Read the model definition and answer for the solid it produces. Units are mm, in the model's axes. Face numbers are marked on the shaded views. A direction names the side the tool comes from. Coordinates: 2 decimals unless noted, no trailing zeros. Write each loop counter-clockwise with the first axis right and the second up, starting at its lowest first coordinate (ties: lowest second). Pieces come first, ordered by that corner, then holes.
Item 1: Section A-A (z = -8.5) is taken. Give the vertices of the cut face in (x, y).
Item 2: Each of these flat-tipped pins is pushed along its axis until it touches: P1, Ø4.5, axis at y = 3.5, z = -5, coming from the +X side; P2, Ø3, axis at x = 11.5, y = 2, coming from the +Z side; P3, Ø2, axis at x = 42, z = 2.5, coming from the -Y side. Where does it stop, or does it pass through?
Item 3: Determine the mould class of the marked faces 4, 5, 6 and 7 for opening direction Y: released by +Y, released by -Y, zero draft, split by the parting line, or undercut.
Item 4: A tool of negligible diameter and unlimited length cuts with its end or side. For the marked faces 1, 2 and 3, from which of +Z, -Z, +X, -X, +Y, -Y can it reach the whole face along a straight path? Write none if from no direction.
Item 5: Section C-C (y = 0) is taken. Give the vertices of the cut face in (x, z).
Item 6: Section D-D (x = 22) is taken. Give the vertices of the cut face in (y, z).
Item 7: Straight lines are drawn through the part: probe 1 along Z at (x, y) = (36.2, 4.75); probe 2 along X at (y, z) = (5.25, -8.25); probe 3 along Z at (x, y) = (16, 1.25). For each, find the intervals that lie inside material, in ascending order.
Item 8: Section B-B (x = 36.2) is taken. Give the vertices of the cut face in (y, z), then the cut area to 3 significant figures.
from build123d import *

# Parameters (mm, degrees)
SKETCH1_W           = 21
SKETCH1_H           = 15.4
BOSS_EXTRUDE1_DEPTH = 40
SKETCH2_W           = 14
SKETCH2_H           = 10
CUT_EXTRUDE1_DEPTH  = 0.5
SKETCH3_W           = 12
SKETCH3_H           = 6.8
CUT_EXTRUDE2_DEPTH  = 0.5
CUT_EXTRUDE3_START  = -15.4
SKETCH3_2_W         = 12
SKETCH3_2_H         = 6.8
CUT_EXTRUDE3_DEPTH  = 0.5
M3_TAPPED_HOLE1_D   = 2.5
M3_TAPPED_HOLE2_D   = 2.5
SKETCH8_R           = 6.4
BOSS_EXTRUDE3_DEPTH = 5
SKETCH9_R           = 3
BOSS_EXTRUDE4_DEPTH = 5
SKETCH10_R          = 2
BOSS_EXTRUDE5_DEPTH = 10
CHAMFER1_SIZE       = 0.4
CHAMFER2_SIZE       = 0.6


with BuildPart() as part:
    # Sketch1 → Boss-Extrude1 (new body)
    with BuildSketch(Plane(origin=(0, 0, 0), x_dir=(0, 0, -1), z_dir=(1, 0, 0))):
        Rectangle(SKETCH1_W, SKETCH1_H)
    extrude(amount=BOSS_EXTRUDE1_DEPTH)

    # Sketch2 → Cut-Extrude1 (cut)
    with BuildSketch(Plane.XY.offset(10.5)):
        with Locations((10.5, 0)):
            Rectangle(SKETCH2_W, SKETCH2_H)
    extrude(amount=-CUT_EXTRUDE1_DEPTH, mode=Mode.SUBTRACT)

    # Sketch3 → Cut-Extrude2 (cut)
    with BuildSketch(Plane(origin=(0, 7.7, 0), x_dir=(1, 0, 0), z_dir=(0, 1, 0))):
        with Locations((26, 7.1)):
            Rectangle(SKETCH3_W, SKETCH3_H)
    extrude(amount=-CUT_EXTRUDE2_DEPTH, mode=Mode.SUBTRACT)

    # Sketch3<2> → Cut-Extrude3 (cut)
    with BuildSketch(Plane(origin=(0, 7.7, 0), x_dir=(1, 0, 0), z_dir=(0, 1, 0)).offset(CUT_EXTRUDE3_START)):
        with Locations((26, 7.1)):
            Rectangle(SKETCH3_2_W, SKETCH3_2_H)
    extrude(amount=CUT_EXTRUDE3_DEPTH, mode=Mode.SUBTRACT)

    # M3 Tapped Hole1 (through all)
    with Locations(Plane(origin=(0, 7.7, 0), x_dir=(-1, 0, 0), z_dir=(0, 1, 0))):
        with Locations((-36.2, -8.5)):
            Hole(M3_TAPPED_HOLE1_D / 2)

    # M3 Tapped Hole2 (through all)
    with Locations(Plane(origin=(0, 7.7, 0), x_dir=(-1, 0, 0), z_dir=(0, 1, 0))):
        with Locations((-16, -8.5)):
            Hole(M3_TAPPED_HOLE2_D / 2)

    # Sketch8 → Boss-Extrude3 (add)
    with BuildSketch(Plane(origin=(40, 0, 0), x_dir=(0, 0, -1), z_dir=(1, 0, 0))):
        Circle(SKETCH8_R)
    extrude(amount=BOSS_EXTRUDE3_DEPTH)

    # Sketch9 → Boss-Extrude4 (add)
    with BuildSketch(Plane(origin=(45, 0, 0), x_dir=(0, 0, -1), z_dir=(1, 0, 0))):
        Circle(SKETCH9_R)
    extrude(amount=BOSS_EXTRUDE4_DEPTH)

    # Sketch10 → Boss-Extrude5 (add)
    with BuildSketch(Plane(origin=(50, 0, 0), x_dir=(0, 0, -1), z_dir=(1, 0, 0))):
        Circle(SKETCH10_R)
    extrude(amount=BOSS_EXTRUDE5_DEPTH)

    # Chamfer1
    chamfer1_edges = [part.edges().sort_by_distance(p)[0] for p in [
        (40, -7.7, 0),
        (10, 7.7, -10.5),
        (40, 0, -10.5),
        (10, -7.7, -10.5),
        (0, -7.7, 0),
        (0, 7.7, 0),
        (0, 0, -10.5),
        (40, 7.7, 0),
        (36, -7.7, -10.5),
        (36, 7.7, -10.5),
    ]]
    chamfer(chamfer1_edges, length=CHAMFER1_SIZE)

    # Chamfer2
    chamfer2_edges = [part.edges().sort_by_distance(p)[0] for p in [
        (40, 0, 10.5),
        (0, 0, 10.5),
        (20, -7.7, 10.5),
        (20, 7.7, 10.5),
        (0.2, -7.5, 10.5),
        (0.2, 7.5, 10.5),
        (39.8, -7.5, 10.5),
        (39.8, 7.5, 10.5),
    ]]
    chamfer(chamfer2_edges, length=CHAMFER2_SIZE)


solid = part.part
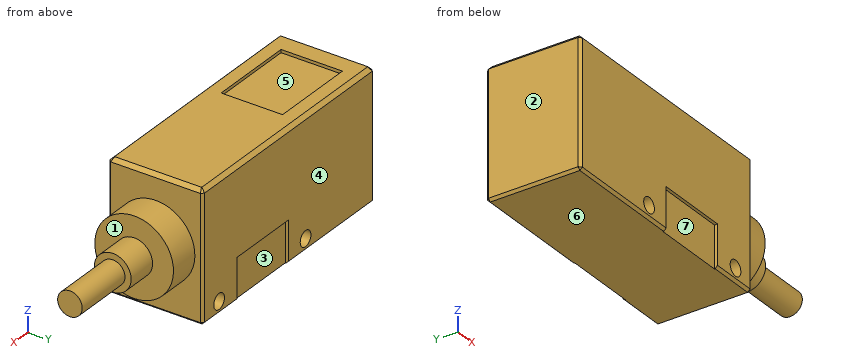
Established:
1. outline: (0, -7.3) - (0.4, -7.7) - (14.75, -7.7) - (14.75, 7.7) - (0.4, 7.7) - (0, 7.3) - close; (17.25, -7.7) - (20, -7.7) - (20, -7.2) - (32, -7.2) - (32, -7.7) - (34.95, -7.7) - (34.95, 7.7) - (32, 7.7) - (32, 7.2) - (20, 7.2) - (20, 7.7) - (17.25, 7.7) - close; (37.45, -7.7) - (39.6, -7.7) - (40, -7.3) - (40, 7.3) - (39.6, 7.7) - (37.45, 7.7) - close
2. P1: stops at x = 45
2. P2: stops at z = 10
2. P3: stops at y = -6.22
3. face 4: released by +Y
3. face 5: undercut
3. face 6: zero draft
3. face 7: released by -Y
4. face 1: +X
4. face 2: +Z, -Z, -X, +Y, -Y
4. face 3: -Z, +Y
5. outline: (0, -10.1) - (0.4, -10.5) - (39.6, -10.5) - (40, -10.1) - (40, -6.4) - (45, -6.4) - (45, -3) - (50, -3) - (50, -2) - (60, -2) - (60, 2) - (50, 2) - (50, 3) - (45, 3) - (45, 6.4) - (40, 6.4) - (40, 9.9) - (39.4, 10.5) - (17.5, 10.5) - (17.5, 10) - (3.5, 10) - (3.5, 10.5) - (0.6, 10.5) - (0, 9.9) - close; hole circle Ø2.5 at (16, -8.5); hole circle Ø2.5 at (36.2, -8.5)
6. outline: (-7.7, -3.7) - (-7.2, -3.7) - (-7.2, -10.5) - (7.2, -10.5) - (7.2, -3.7) - (7.7, -3.7) - (7.7, 9.9) - (7.1, 10.5) - (-7.1, 10.5) - (-7.7, 9.9) - close
7. probe 1: z = -10.5 to -9.75, -7.25 to 10.5
7. probe 2: x = 0 to 14.78, 17.22 to 34.98, 37.42 to 40
7. probe 3: z = -10.5 to -9.75, -7.25 to 10
8. outline: (-7.7, -10.1) - (-7.3, -10.5) - (7.3, -10.5) - (7.7, -10.1) - (7.7, -9.75) - (-7.7, -9.75) - close; (-7.7, -7.25) - (7.7, -7.25) - (7.7, 9.9) - (7.1, 10.5) - (-7.1, 10.5) - (-7.7, 9.9) - close
8. area: 284 mm2
